Geometry check sheet. Reference: drawing and pictorial views, mm from the part's lowest x, y, z. A direction names the side the tool comes from. Give positions to 0.01 mm unless a question says otherwise; leave off trailing zeros. Order: outer loops, then holes, each group sorted by start corner. A loop starts at its lowest first (then second) coordinate and runs counter-clockwise, first axis right, second up.
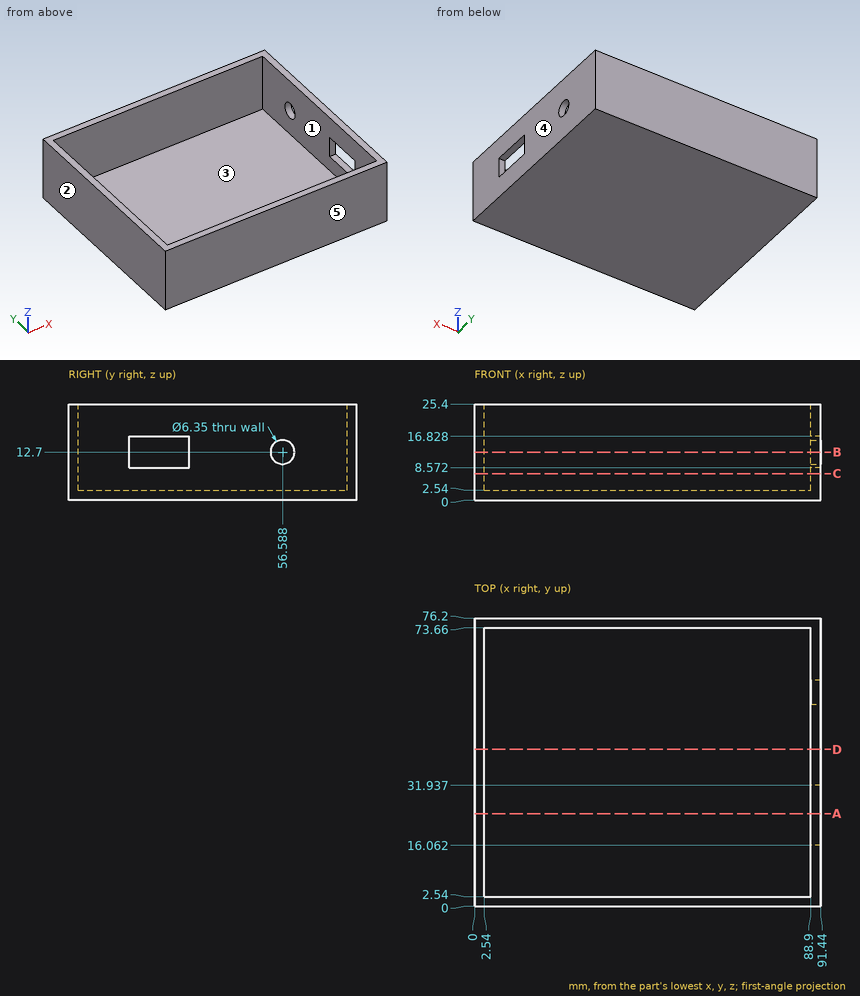
(1) Cross-section at A-A on y = 24.5. Enter the section's corners in (x, z).
Response values:
outline: (0, 0) - (91.44, 0) - (91.44, 8.57) - (88.9, 8.57) - (88.9, 2.54) - (2.54, 2.54) - (2.54, 25.4) - (0, 25.4) - close; (88.9, 16.83) - (91.44, 16.83) - (91.44, 25.4) - (88.9, 25.4) - close
(2) Set-up check for the marked faces 1 and 2: record each of +Z, -Z, +X, -X, +Y, -Y from which the full face is reachable in a straight line by a thin tool's end or side.
Response values:
face 1: +Z
face 2: +Z, -Z, -X, +Y, -Y
(3) Cross-section at B-B on z = 12.7. Enter the section's corners in (x, y).
Response values:
outline: (0, 0) - (91.44, 0) - (91.44, 16.06) - (88.9, 16.06) - (88.9, 2.54) - (2.54, 2.54) - (2.54, 73.66) - (88.9, 73.66) - (88.9, 59.76) - (91.44, 59.76) - (91.44, 76.2) - (0, 76.2) - close; (88.9, 31.94) - (91.44, 31.94) - (91.44, 53.41) - (88.9, 53.41) - close
(4) Release check for a two-part mould opening along Y. For the marked faces 3, 4 and 5 record: released by +Y, released by -Y, zero draft, split by the parting line, or undercut.
Response values:
face 3: undercut
face 4: zero draft
face 5: released by -Y
(5) Material ranges on L1, parallel to X at y = 69.5, z = 16; L2, parallel to Y at x = 60, z = 2.75; L3, parallel to Z at x = 32, y = 16, recorded low to high.
Response values:
L1: x = 0 to 2.54, 88.9 to 91.44
L2: y = 0 to 2.54, 73.66 to 76.2
L3: z = 0 to 2.54
(6) Cross-section at D-D on y = 41.5. Enter the section's corners in (x, z).
Response values:
outline: (0, 0) - (91.44, 0) - (91.44, 25.4) - (88.9, 25.4) - (88.9, 2.54) - (2.54, 2.54) - (2.54, 25.4) - (0, 25.4) - close
(7) Gauge pin test, flat ends, axial feed: pin 1 Ø7 at (y, z) = (24.5, 13) entering from +X; pin 2 Ø4 at (x, y) = (68.5, 39.5) entering from +Z. Record the tip position at first contact, or that the pin passes through.
Response values:
pin 1: stops at x = 2.54
pin 2: stops at z = 2.54
(8) Cross-section at C-C on z = 7. Enter the section's corners in (x, y).
Response values:
outline: (0, 0) - (91.44, 0) - (91.44, 76.2) - (0, 76.2) - close; hole (2.54, 2.54) - (88.9, 2.54) - (88.9, 73.66) - (2.54, 73.66) - close
